from build123d import *

# Parameters (mm, degrees)
F0_R     = 2.25
F0_R_2   = 4.2
F1_DEPTH = 8
F2_DEPTH = 3
F3_W     = 7.4
F3_H     = 7.4
F3_R     = 2.25
F4_DEPTH = 2.4
F5_SIZE  = 1.2


with BuildPart() as f1:
    # F0 (on Top) → F1 (new body)
    with BuildSketch(Plane.XY):
        Polygon((34.5, 5.5), (-5.5, 5.5), (-5.5, -34.5), (3.5, -34.5), (3.5, -3.5), (34.5, -3.5), align=None)
        with Locations((0.45, -28.5)):
            Circle(F0_R, mode=Mode.SUBTRACT)
        Circle(F0_R_2, mode=Mode.SUBTRACT)
        with Locations((28.5, -0.45)):
            Circle(F0_R, mode=Mode.SUBTRACT)
    extrude(amount=F1_DEPTH)

    # F0 (on Top) → F2 (join)
    with BuildSketch(Plane.XY):
        Polygon((3.5, -34.5), (34.5, -3.5), (3.5, -3.5), align=None)
        Circle(F0_R_2)
        Circle(F0_R, mode=Mode.SUBTRACT)
    extrude(amount=F2_DEPTH)

    # F3 (on face) → F4 (cut)
    with BuildSketch(Plane(origin=(0, 0, 0), x_dir=(1, 0, 0), z_dir=(0, 0, -1))):
        with Locations((0.45, 28.5)):
            Rectangle(F3_W, F3_H)
        with Locations((0.45, 28.5)):
            Circle(F3_R, mode=Mode.SUBTRACT)
        with Locations((28.5, 0.45)):
            Rectangle(F3_W, F3_H)
        with Locations((28.5, 0.45)):
            Circle(F3_R, mode=Mode.SUBTRACT)
    extrude(amount=-F4_DEPTH, mode=Mode.SUBTRACT)

    # F5
    f5_edges = [f1.edges().sort_by_distance(p)[0] for p in [
        (-5.5, 5.5, 4),
        (-5.5, -34.5, 4),
        (34.5, 5.5, 4),
        (14.5, 5.5, 8),
        (-5.5, -14.5, 8),
        (-1, -34.5, 8),
        (34.5, 1, 8),
    ]]
    chamfer(f5_edges, length=F5_SIZE)


solid = f1.part
Geometry check sheet. Reference: the model listing, model coordinates, mm. A direction names the side the tool comes from. Coordinates: 2 decimals unless noted, no trailing zeros. Write each loop counter-clockwise with the first axis right and the second up, starting at its lowest first coordinate (ties: lowest second). Pieces come first, ordered by that corner, then holes. Notation, with made-up numbers: (37, 27.5) -> (67, 27.5) arc R12 ccw to (67, 34.5) -> close; hole circle Ø10 at (68, 60.5). An arc over 180 degrees is marked (long way). One line per question, with ' | ' between items.
1. Cross-section at C-C on z = 1.5. Record the cut outline in (x, y).
Answers:
outline: (-5.5, -33.3) -> (-4.3, -34.5) -> (3.5, -34.5) -> (34.5, -3.5) -> (34.5, 4.3) -> (33.3, 5.5) -> (-4.3, 5.5) -> (-5.5, 4.3) -> close; hole (-3.25, -32.2) -> (4.15, -32.2) -> (4.15, -24.8) -> (-3.25, -24.8) -> close; hole circle Ø4.5 at (0, 0); hole (24.8, -4.15) -> (32.2, -4.15) -> (32.2, 3.25) -> (24.8, 3.25) -> close
2. Cross-section at A-A on x = 28.5. Record the cut outline in (y, z), and give its area (3 significant figures).
Answers:
outline: (-9.5, 0) -> (-4.15, 0) -> (-4.15, 2.4) -> (-2.7, 2.4) -> (-2.7, 8) -> (-3.5, 8) -> (-3.5, 3) -> (-9.5, 3) -> close; (1.8, 2.4) -> (3.25, 2.4) -> (3.25, 0) -> (5.5, 0) -> (5.5, 6.8) -> (4.3, 8) -> (1.8, 8) -> close | area: 46.3 mm²
3. Draft check along X on faces 5 (the cylindrical face through (-0.29, 2.23, 1.48)), 6 (the flat face through (0, -24.8, 1)), 7 (the flat face through (-5.5, -14, 3)), 8 (the flat face through (19, -3.5, 5)). Enter one of: +X half, -X half, draft (parallel to the pull), parting line (faces both ways), or undercut.
Answers:
face 5: undercut | face 6: undercut | face 7: -X half | face 8: draft
4. Thickness scan on probe 1 along Y at (x, z) = (0, 1.65); probe 2 along Y at (x, z) = (28.5, 5.7); probe 3 along Y at (x, z) = (0, 7). Record the ranges inside material, lowest first. Write a range as from..to.
Answers:
probe 1: y = -34.5..-32.2, -24.8..-2.25, 2.25..5.5 | probe 2: y = -3.5..-2.7, 1.8..5.5 | probe 3: y = -34.3..-30.7, -26.3..-4.2, 4.2..5.3
5. Set-up check for faces 1 (the flat face through (15, -15, 3)), 2 (the flat face through (15, 5.5, 3)), 3 (the flat face through (24.8, 0, 1)), 4 (the flat face through (2, -2, 3)): record each of +Z, -Z, +X, -X, +Y, -Y from which the full face is reachable in a straight line by a thin tool's end or side.
Answers:
face 1: +Z, +X, -Y | face 2: +Z, -Z, +X, -X, +Y | face 3: -Z | face 4: +Z
6. Cross-section at D-D on x = 15.5. Record the cut outline in (y, z), and give its area (3 significant figures).
Answers:
outline: (-22.5, 0) -> (5.5, 0) -> (5.5, 6.8) -> (4.3, 8) -> (-3.5, 8) -> (-3.5, 3) -> (-22.5, 3) -> close | area: 128 mm²
7. Cross-section at B-B on y = -28.5. Record the cut outline in (x, z).
Answers:
outline: (-5.5, 0) -> (-3.25, 0) -> (-3.25, 2.4) -> (-1.8, 2.4) -> (-1.8, 8) -> (-4.3, 8) -> (-5.5, 6.8) -> close; (2.7, 2.4) -> (4.15, 2.4) -> (4.15, 0) -> (9.5, 0) -> (9.5, 3) -> (3.5, 3) -> (3.5, 8) -> (2.7, 8) -> close
8. Depth check by flat-ended pin: pin 1 Ø1.9 at (y, z) = (-27, 1.5) entering from +X; pin 2 Ø6 at (x, y) = (0.45, -28.5) entering from -Z; pin 3 Ø6.5 at (x, y) = (0, 0) entering from +Z. Enter the tip coordinate at first touch or a pass-through.
Answers:
pin 1: stops at x = 11.95 | pin 2: stops at z = 2.4 | pin 3: stops at z = 3
